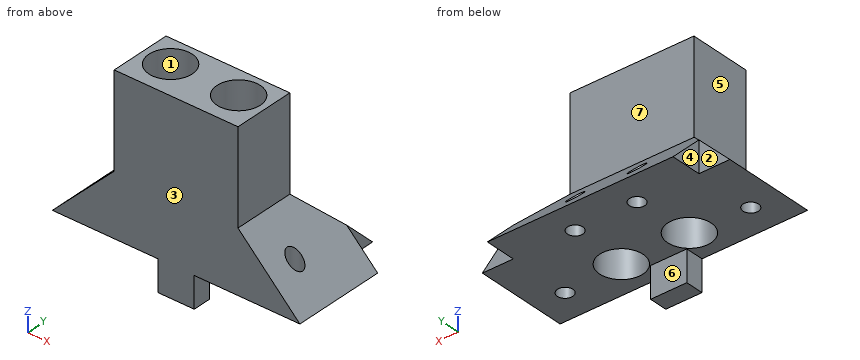
```python
from build123d import *

# Parameters (mm, degrees)
SKETCH_1_W                = 20
SKETCH_1_H                = 20
EXTRUDE_1_DEPTH           = 40
SKETCH_2_W                = 10
SKETCH_2_H                = 15
CUT_EXTRUDE_1_DEPTH       = 7.071067812
PATTERN_CIRCULAR_1_COUNT  = 4
SKETCH_5_R                = 3.5
CUT_EXTRUDE_2_DEPTH       = 25
CUT_EXTRUDE_3_DEPTH       = 5
SKETCH_9_W                = 5.878932188
SKETCH_9_H                = 5.878932188
CUT_EXTRUDE_5_DEPTH       = 5
SKETCH_11_W               = 10
SKETCH_11_H               = 30
EXTRUDE_2_DEPTH           = 10
CUT_EXTRUDE_6_DEPTH       = 30
SKETCH_13_R               = 1.25
CUT_EXTRUDE_7_DEPTH       = 10
PATTERN_CIRCULAR_2_COUNT  = 4
SKETCH_16_W               = 20
SKETCH_16_H               = 10
CUT_EXTRUDE_11_DEPTH      = 40
SKETCH_17_W               = 20
SKETCH_17_H               = 20
SKETCH_17_W_2             = 5.857864376
SKETCH_17_H_2             = 5.857864376
CUT_EXTRUDE_12_DEPTH      = 5
CUT_EXTRUDE_13_DEPTH      = 54.851648071
CUT_EXTRUDE_13_DEPTH_BACK = 10
SKETCH_19_W               = 81.536041923
SKETCH_19_H               = 68.786769913
CUT_EXTRUDE_16_DEPTH      = 400


with BuildPart() as part:
    # 스케치1 → 보스-돌출1 (new body)
    with BuildSketch(Plane.XY):
        Rectangle(SKETCH_1_W, SKETCH_1_H)
    extrude(amount=EXTRUDE_1_DEPTH)

    # 스케치2 → 컷-돌출1 (cut)
    with BuildSketch(Plane(origin=(10, 0, 0), x_dir=(0, 0, -1), z_dir=(1, 0, 0))):
        with Locations((-10, 0)):
            Rectangle(SKETCH_2_W, SKETCH_2_H)
    cut_extrude_1 = extrude(amount=-CUT_EXTRUDE_1_DEPTH, mode=Mode.SUBTRACT)

    # 원형 패턴1: 컷-돌출1 ×4 about axis
    pattern_circular_1_axis = Axis((0, 0, 0), (0, 0, 1))
    for i in range(1, PATTERN_CIRCULAR_1_COUNT):
        add(cut_extrude_1.rotate(pattern_circular_1_axis, i * 360 / PATTERN_CIRCULAR_1_COUNT), mode=Mode.SUBTRACT)

    # 스케치5 → 컷-돌출2 (cut)
    with BuildSketch(Plane.XY.offset(40)):
        with Locations((-5.5, 5.5)):
            Circle(SKETCH_5_R)
        with Locations((5.5, 5.5)):
            Circle(SKETCH_5_R)
        with Locations(Location((-5.5, -5.5, 0), (0, 0, 235.150095421))):
            Circle(SKETCH_5_R)
        with Locations(Location((5.5, -5.5, 0), (0, 0, 304.849904579))):
            Circle(SKETCH_5_R)
    extrude(amount=-CUT_EXTRUDE_2_DEPTH, mode=Mode.SUBTRACT)

    # 스케치6 → 컷-돌출3 (cut)
    with BuildSketch(Plane(origin=(0, 0, 0), x_dir=(-1, 0, 0), z_dir=(0, 0, -1))):
        Polygon((-14.808802863, -2.95), (-14.808802863, 2.95), (-2.95, 2.95), (-2.95, 12.360254216), (2.95, 12.360254216), (2.95, 2.95), (13.852115441, 2.95), (13.852115441, -2.95), (2.95, -2.95), (2.95, -13.975695818), (-2.95, -13.975695818), (-2.95, -2.95), align=None)
    extrude(amount=-CUT_EXTRUDE_3_DEPTH, mode=Mode.SUBTRACT)

    # 스케치9 → 컷-돌출5 (cut)
    with BuildSketch(Plane(origin=(0, 0, 5), x_dir=(-1, 0, 0), z_dir=(0, 0, -1))):
        with Locations((0.010533906, -0.010533906)):
            Rectangle(SKETCH_9_W, SKETCH_9_H)
    extrude(amount=-CUT_EXTRUDE_5_DEPTH, mode=Mode.SUBTRACT)

    # 스케치11 → 보스-돌출2 (add)
    with BuildSketch(Plane(origin=(10, 0, 0), x_dir=(0, 0, -1), z_dir=(1, 0, 0))):
        with Locations((-20, 0)):
            Rectangle(SKETCH_11_W, SKETCH_11_H)
    extrude_2 = extrude(amount=EXTRUDE_2_DEPTH)

    # 스케치12 → 컷-돌출6 (cut)
    with BuildSketch(Plane(origin=(0, 15, 0), x_dir=(1, 0, 0), z_dir=(0, 1, 0))):
        Polygon((20, -15), (10, -25), (20, -25), align=None)
    cut_extrude_6 = extrude(amount=-CUT_EXTRUDE_6_DEPTH, mode=Mode.SUBTRACT)

    # 스케치13 → 컷-돌출7 (cut)
    with BuildSketch(Plane(origin=(0, 0, 15), x_dir=(-1, 0, 0), z_dir=(0, 0, -1))):
        with Locations(Location((-15, -5, 0), (0, 0, 90))):
            Circle(SKETCH_13_R)
        with Locations(Location((-15, 5, 0), (0, 0, 90))):
            Circle(SKETCH_13_R)
    cut_extrude_7 = extrude(amount=-CUT_EXTRUDE_7_DEPTH, mode=Mode.SUBTRACT)

    # 원형 패턴2: 보스-돌출2, 컷-돌출6, 컷-돌출7 ×4 about axis
    pattern_circular_2_axis = Axis((0, 0, 0), (0, 0, 1))
    add([extrude_2.rotate(pattern_circular_2_axis, i * 360 / PATTERN_CIRCULAR_2_COUNT) for i in range(1, PATTERN_CIRCULAR_2_COUNT)])
    add([cut_extrude_6.rotate(pattern_circular_2_axis, i * 360 / PATTERN_CIRCULAR_2_COUNT) for i in range(1, PATTERN_CIRCULAR_2_COUNT)], mode=Mode.SUBTRACT)
    add([cut_extrude_7.rotate(pattern_circular_2_axis, i * 360 / PATTERN_CIRCULAR_2_COUNT) for i in range(1, PATTERN_CIRCULAR_2_COUNT)], mode=Mode.SUBTRACT)

    # 스케치16 → 컷-돌출11 (cut)
    with BuildSketch(Plane.XZ.offset(10)):
        with Locations((0, 5)):
            Rectangle(SKETCH_16_W, SKETCH_16_H)
    extrude(amount=-CUT_EXTRUDE_11_DEPTH, mode=Mode.SUBTRACT)

    # 스케치17 → 컷-돌출12 (cut)
    with BuildSketch(Plane(origin=(0, 0, 10), x_dir=(-1, 0, 0), z_dir=(0, 0, -1))):
        Rectangle(SKETCH_17_W, SKETCH_17_H)
        Rectangle(SKETCH_17_W_2, SKETCH_17_H_2, mode=Mode.SUBTRACT)
    extrude(amount=-CUT_EXTRUDE_12_DEPTH, mode=Mode.SUBTRACT)

    # 스케치18 → 컷-돌출13 (cut, two sides: drawn at the far end of the back side and taken through both)
    with BuildSketch(Plane.XZ.offset(-10).offset(-CUT_EXTRUDE_13_DEPTH_BACK)):
        Polygon((10, 25), (15, 25), (15, 20), align=None)
    extrude(amount=CUT_EXTRUDE_13_DEPTH + CUT_EXTRUDE_13_DEPTH_BACK, mode=Mode.SUBTRACT)

    # 스케치19 → 컷-돌출16 (cut)
    with BuildSketch(Plane(origin=(0, 0, 0), x_dir=(1, 0, 0), z_dir=(0, 1, 0))):
        with Locations((9.636077682, -26.334226141)):
            Rectangle(SKETCH_19_W, SKETCH_19_H)
    extrude(amount=-CUT_EXTRUDE_16_DEPTH, mode=Mode.SUBTRACT)


solid = part.part
```
Geometry: final body of the model. Coordinates: model frame, mm. Face numbers are marked on the shaded views. A direction names the side the tool comes from. Round coordinates to 2 decimals unless told otherwise and drop trailing zeros. Order: outer loops, then holes, each group sorted by start corner. A loop starts at its lowest first (then second) coordinate and runs counter-clockwise, first axis right, second up. Notation, with made-up numbers: (61, -32) - (92, -32) arc R10 ccw to (92, -15) - close; hole circle Ø2 at (75, -22.75). An arc over 180 degrees is marked (long way). Use CSV: the item, a comma, the result in double quotes. Start each with the question number.
Q1. Mould query, pull axis Y, two halves, no side actions, for the marked faces 1, 2 and 3. Classes: +Y half, -Y half, draft (parallel to the pull), parting line (faces both ways), or undercut.
Q2. Material intervals for line 1 along X through (y, z) = (8.5, 22.5); line 2 along Y through (x, z) = (-5, 17.75); line 3 along X through (y, z) = (5, 19.5), sorted ascending. Write a range as from..to.
Q3. Section query D-D (y = 5.5). Return loops of the section in (x, z), and give its area (3 significant figures).
Q4. Section query C-C (z = 36.25). Return loops of the section in (x, y).
Q5. First-contact query: pin 1 (3 mm diameter, centred on x = -15, z = 17, fed in from +Y); pin 2 (2.5 mm diameter, centred on y = 2, z = 11.5, fed in from -X); pin 3 (1.5 mm diameter, centred on x = 16, y = 7, fed in from +Z). Flat tips, straight axial feed; report the tip coordinate or a pass-through.
Q6. Section query B-B (x = -8). Return loops of the section in (y, z).
Q7. Access query for the marked faces 4, 5, 6 and 7. Directions: +Z, -Z, +X, -X, +Y, -Y. A direction counts if a zero-diameter tool reaches every point of the face in a straight line with its end or side. Return the directions, or none.
Q8. Section query A-A (y = 15.75). Return loops of the section in (x, z).
Result set:
1,face 1,"undercut"
1,face 2,"+Y half"
1,face 3,"-Y half"
2,line 1,"x = -12.5..-7.3, -3.7..3.7, 7.3..12.5"
2,line 2,"y = 0..2.04, 8.96..13.75, 16.25..17.25"
2,line 3,"x = -13.75..-8.96, -2.04..2.04, 8.96..13.75"
3,outline,"(-20, 15) - (-16.15, 15) - (-16.15, 18.85) - close; (-13.85, 15) - (-9, 15) - (-9, 40) - (-10, 40) - (-10, 25) - (-13.85, 21.15) - close; (-2, 15) - (2, 15) - (2, 40) - (-2, 40) - close; (9, 15) - (13.85, 15) - (13.85, 21.15) - (10, 25) - (10, 40) - (9, 40) - close; (16.15, 15) - (20, 15) - (16.15, 18.85) - close"
3,area,"227 mm2"
4,outline,"(-10, 0) - (10, 0) - (10, 10) - (-10, 10) - close; hole circle Ø7 at (-5.5, 5.5); hole circle Ø7 at (5.5, 5.5)"
5,pin 1,"stops at y = 19.5"
5,pin 2,"stops at x = -2.93"
5,pin 3,"stops at z = 19.75"
6,outline,"(0, 15) - (3.05, 15) - (3.05, 40) - (0, 40) - close; (7.95, 15) - (20, 15) - (10, 25) - (10, 40) - (7.95, 40) - close"
7,face 4,"+Z, -Z, -X, +Y"
7,face 5,"+Z, -X, +Y, -Y"
7,face 6,"-Z, +X, -X, +Y"
7,face 7,"+Z, +X, -X, +Y"
8,outline,"(-15, 15) - (-6, 15) - (-6, 19.25) - (-15, 19.25) - close; (-4, 15) - (4, 15) - (4, 19.25) - (-4, 19.25) - close; (6, 15) - (15, 15) - (15, 19.25) - (6, 19.25) - close"
